Geometry check sheet. Reference: drawing and pictorial views, mm from the part's lowest x, y, z. A direction names the side the tool comes from. Give positions to 0.01 mm unless a question says otherwise; leave off trailing zeros. Loops run counter-clockwise (first coordinate to the right, second up) from the corner with the lowest first, then second, coordinate; pieces in that order, holes last. Notation, with made-up numbers: (-31, -15) - (-25, -15) arc R24 ccw to (-25, 12) - close; hole circle Ø8 at (49, 72.5). An arc over 180 degrees is marked (long way). Answer in a Markdown table with one row per item. Add a question column.
(1) Sectioned sample at B-B on x = 3. Enter the section's corners in (y, z).
(2) Thickness scan on L1, parallel to Y at x = 3, z = 2.1; L2, parallel to Z at x = 2.45, y = 4.5; L3, parallel to Z at x = 3.75, y = 3.65. Record the ranges inside material, lowest first.
(3) Sectioned sample at D-D on z = 8. Enter the section's corners in (x, y).
(4) Go/stop test with flat-tipped pins: P1, Ø1.5, axis at x = 2.5, y = 3, coming from the -Z side; P2, Ø3, axis at x = 5, y = 3.5, coming from the +Z side. Record where each tip stops, or that it passes through.
(5) Set-up check for the marked faces 1 and 2: record each of +Z, -Z, +X, -X, +Y, -Y from which the full face is reachable in a straight line by a thin tool's end or side.
(6) Sectioned sample at A-A on z = 2.5. Enter the section's corners in (x, y).
(7) Sectioned sample at C-C on y = 1.45. Enter the section's corners in (x, z) (1 decimal).
(8) Draft check along Y on the marked faces 3, 4 and 5. Enter one of: released by +Y, released by -Y, zero draft, split by the parting line, or undercut.
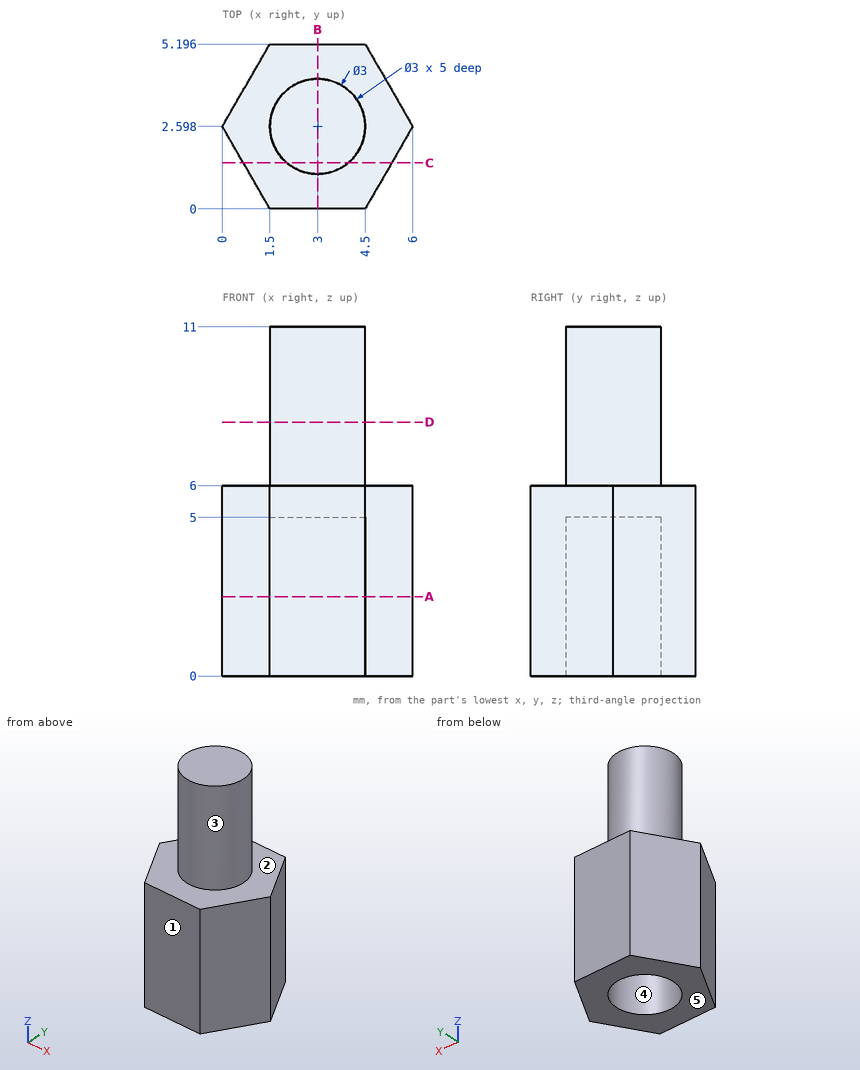
Reply:
| question | item | result |
|---|---|---|
| 1 | outline | (0, 0) - (1.1, 0) - (1.1, 5) - (4.1, 5) - (4.1, 0) - (5.2, 0) - (5.2, 6) - (4.1, 6) - (4.1, 11) - (1.1, 11) - (1.1, 6) - (0, 6) - close |
| 2 | L1 | 0 to 1.1, 4.1 to 5.2 |
| 2 | L2 | 0 to 6 |
| 2 | L3 | 5 to 11 |
| 3 | outline | circle Ø3 at (3, 2.6) |
| 4 | P1 | z = 5 |
| 4 | P2 | z = 11 |
| 5 | face 1 | +Z, -Z, +X, -X, -Y |
| 5 | face 2 | +Z |
| 6 | outline | (0, 2.6) - (1.5, 0) - (4.5, 0) - (6, 2.6) - (4.5, 5.2) - (1.5, 5.2) - close; hole circle Ø3 at (3, 2.6) |
| 7 | outline | (0.7, 0) - (2, 0) - (2, 5) - (4, 5) - (4, 0) - (5.3, 0) - (5.3, 6) - (4, 6) - (4, 11) - (2, 11) - (2, 6) - (0.7, 6) - close |
| 8 | face 3 | split by the parting line |
| 8 | face 4 | undercut |
| 8 | face 5 | zero draft |
